from build123d import *

# Parameters (mm, degrees)
AUFSATZ_LINEAR_AUSTRAGEN1_DEPTH    = 10
F_10_0_10_DURCHMESSER_BOHRUNG1_D   = 10
SKIZZE8_W                          = 43
SKIZZE8_H                          = 43
SCHNITT_LINEAR_AUSTRAGEN2_DEPTH    = 10
M3_GEWINDEBOHRUNG1_D               = 2.5
M3_GEWINDEBOHRUNG1_DEPTH           = 8
M3_GEWINDEBOHRUNG1_CSINK_D         = 3.05
M3_GEWINDEBOHRUNG1_CSINK_ANGLE     = 90
M3_GEWINDEBOHRUNG1_TIP             = 0.751075774
F_5_0_5_DURCHMESSER_BOHRUNG1_D     = 5
DURCHGANGSLOCH_F_R_M101_AT_2_COUNT = 2
DURCHGANGSLOCH_F_R_M101_AT_2_PITCH = 70
DURCHGANGSLOCH_F_R_M101_AT_3_COUNT = 2
DURCHGANGSLOCH_F_R_M101_AT_3_PITCH = 50
DURCHGANGSLOCH_F_R_M101_AT_4_COUNT = 2
DURCHGANGSLOCH_F_R_M101_AT_4_PITCH = 86.02325267


with BuildPart() as part:
    # Skizze1 → Aufsatz-Linear austragen1 (new body)
    with BuildSketch(Plane(origin=(0, 0, 0), x_dir=(1, 0, 0), z_dir=(0, 1, 0))):
        with BuildLine():
            Line((-105, 90), (105, 90))
            ThreePointArc((105, 90), (112.071067812, 87.071067812), (115, 80))
            Line((115, 80), (115, 50))
            ThreePointArc((115, 50), (112.071067812, 42.928932188), (105, 40))
            Line((105, 40), (55, 40))
            ThreePointArc((55, 40), (44.393398282, 35.606601718), (40, 25))
            Line((40, 25), (40, -45))
            ThreePointArc((40, -45), (44.393398282, -55.606601718), (55, -60))
            Line((55, -60), (65, -60))
            ThreePointArc((65, -60), (72.071067812, -62.928932188), (75, -70))
            Line((75, -70), (75, -80))
            ThreePointArc((75, -80), (72.071067812, -87.071067812), (65, -90))
            Line((65, -90), (-65, -90))
            ThreePointArc((-65, -90), (-72.071067812, -87.071067812), (-75, -80))
            Line((-75, -80), (-75, -70))
            ThreePointArc((-75, -70), (-72.071067812, -62.928932188), (-65, -60))
            Line((-65, -60), (-55, -60))
            ThreePointArc((-55, -60), (-44.393398282, -55.606601718), (-40, -45))
            Line((-40, -45), (-40, 25))
            ThreePointArc((-40, 25), (-44.393398282, 35.606601718), (-55, 40))
            Line((-55, 40), (-105, 40))
            ThreePointArc((-105, 40), (-112.071067812, 42.928932188), (-115, 50))
            Line((-115, 50), (-115, 80))
            ThreePointArc((-115, 80), (-112.071067812, 87.071067812), (-105, 90))
        make_face()
    extrude(amount=AUFSATZ_LINEAR_AUSTRAGEN1_DEPTH)

    # Ø10.0 (10) Durchmesser Bohrung1 (through all)
    with Locations(Plane(origin=(0, 10, 0), x_dir=(1, 0, 0), z_dir=(0, 1, 0))):
        with Locations((-85, 65), (85, 65)):
            Hole(F_10_0_10_DURCHMESSER_BOHRUNG1_D / 2)

    # Skizze8 → Schnitt-Linear austragen2 (cut)
    with BuildSketch(Plane(origin=(0, 10, 0), x_dir=(1, 0, 0), z_dir=(0, 1, 0))):
        with Locations((0, 50)):
            Rectangle(SKIZZE8_W, SKIZZE8_H)
    extrude(amount=-SCHNITT_LINEAR_AUSTRAGEN2_DEPTH, mode=Mode.SUBTRACT)

    # M3 Gewindebohrung1
    with Locations(Plane(origin=(0, 10, 0), x_dir=(1, 0, 0), z_dir=(0, 1, 0))):
        with Locations((-29.5, 79.5), (-29.5, 20.5), (29.5, 20.5), (29.5, 79.5)):
            CounterSinkHole(M3_GEWINDEBOHRUNG1_D / 2, M3_GEWINDEBOHRUNG1_CSINK_D / 2, depth=M3_GEWINDEBOHRUNG1_DEPTH, counter_sink_angle=M3_GEWINDEBOHRUNG1_CSINK_ANGLE)
            with Locations((0, 0, -(M3_GEWINDEBOHRUNG1_DEPTH + M3_GEWINDEBOHRUNG1_TIP / 2))):  # 118° drill point
                Cone(0, M3_GEWINDEBOHRUNG1_D / 2, M3_GEWINDEBOHRUNG1_TIP, mode=Mode.SUBTRACT)

    # Ø5.0 (5) Durchmesser Bohrung1 (through all)
    with Locations(Plane(origin=(0, 0, 0), x_dir=(-1, 0, 0), z_dir=(0, -1, 0))):
        with Locations((77.5, 72.5), (92.5, 57.5), (-92.5, 72.5), (-77.5, 57.5)):
            Hole(F_5_0_5_DURCHMESSER_BOHRUNG1_D / 2)

    # Skizze14 → Durchgangsloch für M101 (revolve, cut)
    with BuildSketch(Plane(origin=(25, 0, 5), x_dir=(0, 0, -1), z_dir=(1, 0, 0))):
        Polygon((0, 0), (0, 10), (7.5, 10), (5.5, 8), (5.5, 0), align=None)
    durchgangsloch_f_r_m101 = revolve(axis=Axis((25, -6.35, 5), (0, 1, 0)), mode=Mode.SUBTRACT)

    # Durchgangsloch für M101 at 2: Durchgangsloch für M101 ×2
    with Locations(*[(0, 0, i * DURCHGANGSLOCH_F_R_M101_AT_2_PITCH) for i in range(1, DURCHGANGSLOCH_F_R_M101_AT_2_COUNT)]):
        add(durchgangsloch_f_r_m101, mode=Mode.SUBTRACT)

    # Durchgangsloch für M101 at 3: Durchgangsloch für M101 ×2
    with Locations(*[(-i * DURCHGANGSLOCH_F_R_M101_AT_3_PITCH, 0, 0) for i in range(1, DURCHGANGSLOCH_F_R_M101_AT_3_COUNT)]):
        add(durchgangsloch_f_r_m101, mode=Mode.SUBTRACT)

    # Durchgangsloch für M101 at 4: Durchgangsloch für M101 ×2
    with Locations(*[Vector(-0.5812381937190965, 0, 0.813733471206735) * (i * DURCHGANGSLOCH_F_R_M101_AT_4_PITCH) for i in range(1, DURCHGANGSLOCH_F_R_M101_AT_4_COUNT)]):
        add(durchgangsloch_f_r_m101, mode=Mode.SUBTRACT)


solid = part.part
Work out the finished part from the listing and answer in its coordinate system (mm). A direction names the side the tool comes from. Coordinates: 2 decimals unless noted, no trailing zeros. Loops run counter-clockwise (first coordinate to the right, second up) from the corner with the lowest first, then second, coordinate; pieces in that order, holes last. Notation, with made-up numbers: (-4, 82) -> (29, 82) arc R20 ccw to (29, 94) -> close; hole circle Ø2 at (12, -4). An arc over 180 degrees is marked (long way). Answer as CSV lines item,"result".
1) The part is cut by section C-C (z = -57.5). Give the vertices of the cut face in (x, y), and give its area (3 significant figures).
A:
outline,"(-115, 0) -> (-95, 0) -> (-95, 10) -> (-115, 10) -> close; (-90, 0) -> (-21.5, 0) -> (-21.5, 10) -> (-90, 10) -> close; (21.5, 0) -> (75, 0) -> (75, 10) -> (21.5, 10) -> close; (80, 0) -> (115, 0) -> (115, 10) -> (80, 10) -> close"
area,"1,770 mm²"
2) Flat-ended cylindrical pins translate along their axes: pin 1 (6.5 mm diameter, centred on x = -25, z = 75, fed in from +Y); pin 2 (3 mm diameter, centred on y = 3, z = 72.5, fed in from -X); pin 3 (3 mm diameter, centred on x = 29.5, z = -20.5, fed in from +Y) (3 decimals); pin 4 (1 mm diameter, centred on y = 1.5, z = 53.5, fed in from -X). Find the tip coordinate at first contact, or state that the pin passes through.
A:
pin 1,"passes through"
pin 2,"stops at x = -75"
pin 3,"stops at y = 9.975"
pin 4,"stops at x = -43"
3) The part is cut by section A-A (x = -14.5). Give the vertices of the cut face in (y, z), and give its area (3 significant figures).
A:
outline,"(0, -90) -> (10, -90) -> (10, -71.5) -> (0, -71.5) -> close; (0, -28.5) -> (10, -28.5) -> (10, 90) -> (0, 90) -> close"
area,"1,370 mm²"
4) For a pull along Z with two mould halves and no side action, classify faces 4 (the face through (115, 5, -65)), 5 (the face through (-112.15, 4.93, -86.99)), 6 (the face through (60, 5, 60)), 7 (the face through (-111.99, 4.93, -42.85)) as released by +Z, released by -Z, zero draft, split by the parting line, or undercut.
A:
face 4,"zero draft"
face 5,"released by -Z"
face 6,"undercut"
face 7,"released by +Z"
5) Straight lines are drawn through the part: probe 1 along Z at (x, y) = (25, 4.75); probe 2 along X at (y, z) = (8, -79.5); probe 3 along X at (y, z) = (4.25, -20.5). For each, find the intervals that lie inside material, in ascending order.
A:
probe 1,"z = -90 to -0.5, 10.5 to 69.5, 80.5 to 90"
probe 2,"x = -115 to -30.75, -28.25 to 28.25, 30.75 to 115"
probe 3,"x = -40 to -30.75, -28.25 to 28.25, 30.75 to 40"
6) For faces 1 (the face through (-44.28, 4.93, -35.49)), 2 (the face through (44.51, 4.93, -35.72)), 3 (the face through (21.5, 5, -50)), determine the directions among +Z, -Z, +X, -X, +Y, -Y from which every point of the face is accessible in a straight line to the end or side of a thin tool.
A:
face 1,"-X, +Y, -Y"
face 2,"+X, +Y, -Y"
face 3,"+Y, -Y"
7) The part is cut by section D-D (x = -43). Give the vertices of the cut face in (y, z), and give its area (3 significant figures).
A:
outline,"(0, -90) -> (10, -90) -> (10, -34) -> (0, -34) -> close; (0, 54) -> (10, 54) -> (10, 90) -> (0, 90) -> close"
area,"920 mm²"
8) The part is cut by section B-B (z = 5). Give the vertices of the cut face in (x, y).
A:
outline,"(-40, 0) -> (-30.5, 0) -> (-30.5, 8) -> (-32.5, 10) -> (-40, 10) -> close; (-19.5, 0) -> (19.5, 0) -> (19.5, 8) -> (17.5, 10) -> (-17.5, 10) -> (-19.5, 8) -> close; (30.5, 0) -> (40, 0) -> (40, 10) -> (32.5, 10) -> (30.5, 8) -> close"
